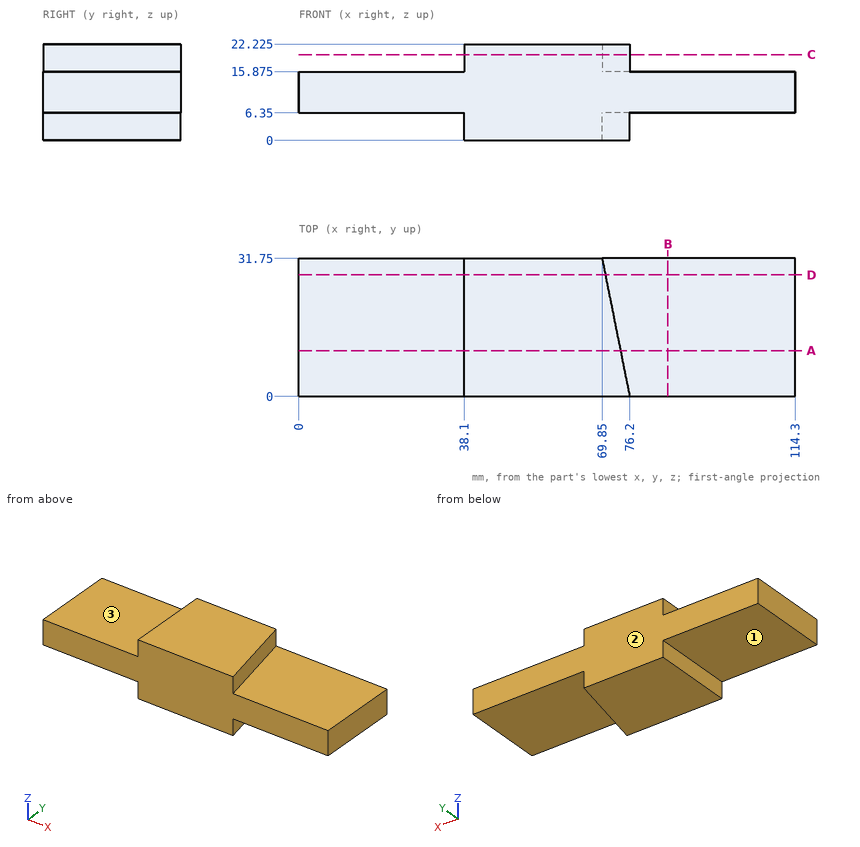
Geometry check sheet. Reference: drawing and pictorial views, mm from the part's lowest x, y, z. A direction names the side the tool comes from. Give positions to 0.01 mm unless a question says otherwise; leave off trailing zeros. Write each loop counter-clockwise with the first axis right and the second up, starting at its lowest first coordinate (ties: lowest second). Pieces come first, ordered by that corner, then holes.
Item 1: Cross-section at D-D (y = 28). Enter the section's corners in (x, z) (3 decimals), and give its area (3 significant figures).
Item 2: Scan lines: L1, parallel to Z at x = 27, y = 9.5 (3 decimals); L2, parallel to X at y = 14, z = 3.5; L3, parallel to X at y = 29, z = 1. Record each from-to range of solid material in increasing order.
Item 3: Cross-section at C-C (z = 19.75). Enter the section's corners in (x, y), and give its area (3 significant figures).
Item 4: Gauge pin test, flat ends, axial feed: pin 1 (9.5 mm diameter, centred on x = 96.5, y = 14.5, fed in from +Z) (3 decimals); pin 2 (4 mm diameter, centred on y = 6, z = 3, fed in from +X); pin 3 (1.9 mm diameter, centred on y = 23, z = 1.5, fed in from -X). Record the tip position at first contact, or that the pin passes through.
Item 5: Cross-section at A-A (y = 10.5). Enter the section's corners in (x, z) (3 decimals), and give its area (3 significant figures).
Item 6: Access from +Z, -Z, +X, -X, +Y, -Y to the whole of each face (thin tool, end or side, straight path). Record for the marked faces 1, 2 and 3.
Item 7: Cross-section at B-B (x = 85). Enter the section's corners in (y, z) (3 decimals).
Report:
1. outline: (0, 6.35) - (38.1, 6.35) - (38.1, 0) - (70.6, 0) - (70.6, 6.35) - (114.3, 6.35) - (114.3, 15.875) - (70.6, 15.875) - (70.6, 22.225) - (38.1, 22.225) - (38.1, 15.875) - (0, 15.875) - close
1. area: 1,500 mm2
2. L1: z = 6.35 to 15.875
2. L2: x = 38.1 to 73.4
2. L3: x = 38.1 to 70.4
3. outline: (38.1, 0) - (76.2, 0) - (69.85, 31.75) - (38.1, 31.75) - close
3. area: 1,110 mm2
4. pin 1: stops at z = 15.875
4. pin 2: stops at x = 75.4
4. pin 3: stops at x = 38.1
5. outline: (0, 6.35) - (38.1, 6.35) - (38.1, 0) - (74.1, 0) - (74.1, 6.35) - (114.3, 6.35) - (114.3, 15.875) - (74.1, 15.875) - (74.1, 22.225) - (38.1, 22.225) - (38.1, 15.875) - (0, 15.875) - close
5. area: 1,550 mm2
6. face 1: -Z, -X, +Y, -Y
6. face 2: +Z, -Z, +X, -X, +Y
6. face 3: +Z, -X, +Y, -Y
7. outline: (0, 6.35) - (31.75, 6.35) - (31.75, 15.875) - (0, 15.875) - close
